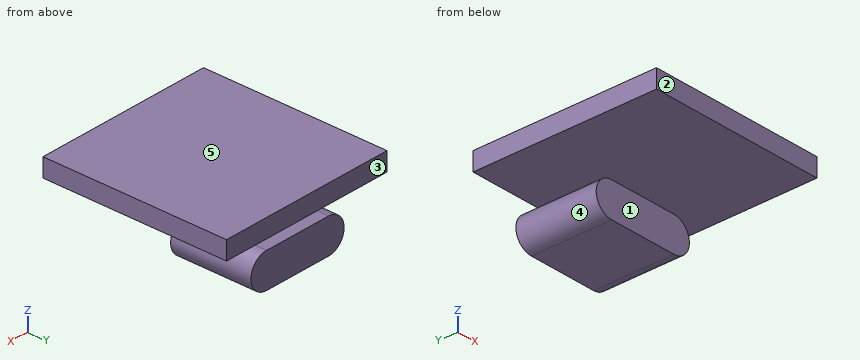
```python
from build123d import *

# Parameters (mm, degrees)
ESBO_O1_W                     = 15.5
ESBO_O1_H                     = 16
RESSALTO_EXTRUS_O1_DEPTH      = 1.6
RESSALTO_EXTRUS_O2_DEPTH      = 1
RESSALTO_EXTRUS_O2_DEPTH_BACK = 6


with BuildPart() as part:
    # Esboço1 → Ressalto-extrusão1 (new body)
    with BuildSketch(Plane.XY):
        Rectangle(ESBO_O1_W, ESBO_O1_H)
    extrude(amount=RESSALTO_EXTRUS_O1_DEPTH)

    # Esboço3 → Ressalto-extrusão2 (add, two sides)
    with BuildSketch(Plane(origin=(0, 8, 0), x_dir=(1, 0, 0), z_dir=(0, 1, 0))) as ressalto_extrus_o2_sk:
        with BuildLine():
            Line((-1, 3), (5, 3))
            ThreePointArc((5, 3), (6.5, 1.5), (5, 0))
            Line((5, 0), (-1, 0))
            ThreePointArc((-1, 0), (-2.5, 1.5), (-1, 3))
        make_face()
    extrude(amount=RESSALTO_EXTRUS_O2_DEPTH)
    extrude(ressalto_extrus_o2_sk.sketch, amount=-RESSALTO_EXTRUS_O2_DEPTH_BACK)


solid = part.part
```
The listing builds one solid part. Answer for the finished solid, in the listing's coordinates (mm). Face numbers are marked on the shaded views. A direction names the side the tool comes from. Coordinates: 2 decimals unless noted, no trailing zeros. Loops run counter-clockwise (first coordinate to the right, second up) from the corner with the lowest first, then second, coordinate; pieces in that order, holes last. Notation, with made-up numbers: M 37.5,-11.75 L 60.5,-11.75 A21 ccw 60.5,19.25 Z; hole C 29.5,79.25 d6. An arc over 180 degrees is marked long. Answer as a JSON object with one key per item and string values. Group by question number.
Item 1: Consider L1, parallel to Y at x = 2.25, z = -1.7; L2, parallel to Z at x = 1.25, y = 0.75; L3, parallel to Y at x = -1.25, z = 1. Determine where each line is inside the solid, lowest interval first.
Item 2: Section A-A (x = 5.5) is taken. Write down the section's boundary in (y, z).
Item 3: Determine the mould class of the marked faces 3, 4 and 5 for opening direction Z: +Z half, -Z half, draft (parallel to the pull), parting line (faces both ways), or undercut.
Item 4: Section D-D (z = 0.7) is taken. Write down the section's boundary in (x, y), and give its area (3 significant figures).
Item 5: Each of these flat-tipped pins is pushed along its axis until it touches: P1, Ø0.9, axis at x = 1, z = -2, coming from the -Y side; P2, Ø0.5, axis at x = 1, y = 8.5, coming from the +Z side; P3, Ø1.5, axis at y = 5, z = -0.5, coming from the +X side. Where does it stop, or does it pass through?
Item 6: Which of the six approach directions +Z, -Z, +X, -X, +Y, -Y give full straight-line access (tool end or side, diameter ignored) to the marked faces 1 and 2?
Item 7: Section B-B (y = 5) is taken. Write down the section's boundary in (x, z), and give its area (3 significant figures).
Item 8: Section C-C (x = 2.5) is taken. Write down the section's boundary in (y, z).
Solved:
{
 "1": {"L1": "y = 2 to 9", "L2": "z = 0 to 1.6", "L3": "y = -8 to 8"},
 "2": {"outline": "M -8,0 L 8,0 L 8,1.6 L -8,1.6 Z; M 2,-2.91 L 9,-2.91 L 9,-0.09 L 2,-0.09 Z"},
 "3": {"face 3": "draft", "face 4": "undercut", "face 5": "+Z half"},
 "4": {"outline": "M -7.75,-8 L 7.75,-8 L 7.75,8 L -7.75,8 Z", "area": "248 mm2"},
 "5": {"P1": "stops at y = 2", "P2": "stops at z = 0", "P3": "stops at x = 7.75"},
 "6": {"face 1": "-Z, +X, -X, -Y", "face 2": "+Z, -Z, +X, -X, -Y"},
 "7": {"outline": "M -7.75,0 L -1,0 A1.5 ccw -1,-3 L 5,-3 A1.5 ccw 5,0 L 7.75,0 L 7.75,1.6 L -7.75,1.6 Z", "area": "49.9 mm2"},
 "8": {"outline": "M -8,0 L 2,0 L 2,-3 L 9,-3 L 9,0 L 8,0 L 8,1.6 L -8,1.6 Z"}
}
